Part model, mm, in its own coordinate system. Round coordinates to 2 decimals unless told otherwise and drop trailing zeros. Loops run counter-clockwise (first coordinate to the right, second up) from the corner with the lowest first, then second, coordinate; pieces in that order, holes last.
1) Drop flat-ended pins along their axis: P1, Ø2.5, axis at x = -4.19, y = 5.62, coming from the +Z side; P2, Ø0.6, axis at y = 1.5, z = 0.5, coming from the -X side. Give the stop position or say it passes through.
2) Probe line 1 (X direction, y = 6, z = 0.9); line 2 (Y direction, x = 2.25, z = 0.2); line 3 (Y direction, x = -4.75, z = 0.3). List the from-to ranges inside material, lowest first.
3) Band-saw the part on B-B, the plane z = 0.8. State how many separate pieces and enclosed holes the cut face has, then the cut area to 3 significant figures.
4) Band-saw the part on A-A, the plane x = 0. Write the cut outline in (y, z).
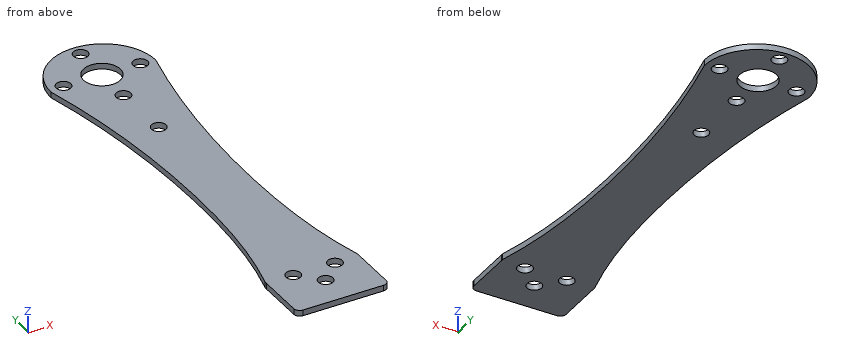
from build123d import *

# Parameters (mm, degrees)
BOSS_EXTRUDE1_DEPTH = 1.27
SKETCH3_R           = 1.5875
SKETCH3_R_2         = 3.9878
CUT_EXTRUDE1_DEPTH  = 97.298395578


with BuildPart() as part:
    # Sketch1 → Boss-Extrude1 (new body)
    with BuildSketch(Plane.XY):
        with BuildLine():
            Line((10.0076, 5.622584698), (10.0076, -4.7117))
            ThreePointArc((10.0076, -4.7117), (9.635625612, -5.609725612), (8.7376, -5.9817))
            Line((8.7376, -5.9817), (-8.7376, -5.9817))
            ThreePointArc((-8.7376, -5.9817), (-9.635625612, -5.609725612), (-10.0076, -4.7117))
            Line((-10.0076, -4.7117), (-10.0076, 5.622584698))
            ThreePointArc((-10.0076, 5.622584698), (-10.003391038, 5.85374719), (-9.990769733, 6.084603239))
            add(Edge.make_bspline(
                [(-9.990769733, 6.084603239), (-7.167817584, 16.591535459), (-5.051519119, 42.938826991), (-7.717998868, 69.224459282), (-11.3538, 84.2645)],
                knots=[0, 0, 0, 0, 0.412468481, 1, 1, 1, 1], degree=3))
            ThreePointArc((-11.3538, 84.2645), (0, 95.6183), (11.3538, 84.2645))
            add(Edge.make_bspline(
                [(9.990769733, 6.084603239), (7.167817584, 16.591535459), (5.051519119, 42.938826991), (7.717998868, 69.224459282), (11.3538, 84.2645)],
                knots=[0, 0, 0, 0, 0.412468481, 1, 1, 1, 1], degree=3))
            ThreePointArc((9.990769733, 6.084603239), (10.003391038, 5.85374719), (10.0076, 5.622584698))
        make_face()
    extrude(amount=BOSS_EXTRUDE1_DEPTH)

    # Sketch3 → Cut-Extrude1 (cut, through all)
    with BuildSketch(Plane.XY.offset(1.27)):
        with Locations((0.009537188, 63.488174324)):
            Circle(SKETCH3_R)
        with Locations((-4.18787141, 5.623885886)):
            Circle(SKETCH3_R)
        with Locations((0.009537188, 84.824174324)):
            Circle(SKETCH3_R_2)
        with Locations((4.790889658, 5.460027166)):
            Circle(SKETCH3_R)
        with Locations((0.219579764, 1.052575992)):
            Circle(SKETCH3_R)
        with Locations((8.263377785, 84.685825499)):
            Circle(SKETCH3_R)
        with Locations((-0.117124746, 76.531516693)):
            Circle(SKETCH3_R)
        with Locations((-8.243855334, 84.987075758)):
            Circle(SKETCH3_R)
        with Locations((0.160867255, 93.116418474)):
            Circle(SKETCH3_R)
    extrude(amount=-CUT_EXTRUDE1_DEPTH, mode=Mode.SUBTRACT)


solid = part.part
Reported:
1. P1: passes through
1. P2: stops at x = -10.01
2. line 1: x = -10 to -5.73, -2.65 to 3.3, 6.28 to 10
2. line 2: y = -5.98 to 81.53, 88.12 to 95.39
2. line 3: y = -5.98 to 4.14, 7.11 to 94.58
3. separate pieces: 1
3. enclosed holes: 9
3. area: 1,530 mm2
4. outline: (-5.98, 0) - (-0.52, 0) - (-0.52, 1.27) - (-5.98, 1.27) - close; (2.62, 0) - (61.9, 0) - (61.9, 1.27) - (2.62, 1.27) - close; (65.08, 0) - (74.95, 0) - (74.95, 1.27) - (65.08, 1.27) - close; (78.11, 0) - (80.84, 0) - (80.84, 1.27) - (78.11, 1.27) - close; (88.81, 0) - (91.54, 0) - (91.54, 1.27) - (88.81, 1.27) - close; (94.7, 0) - (95.62, 0) - (95.62, 1.27) - (94.7, 1.27) - close
